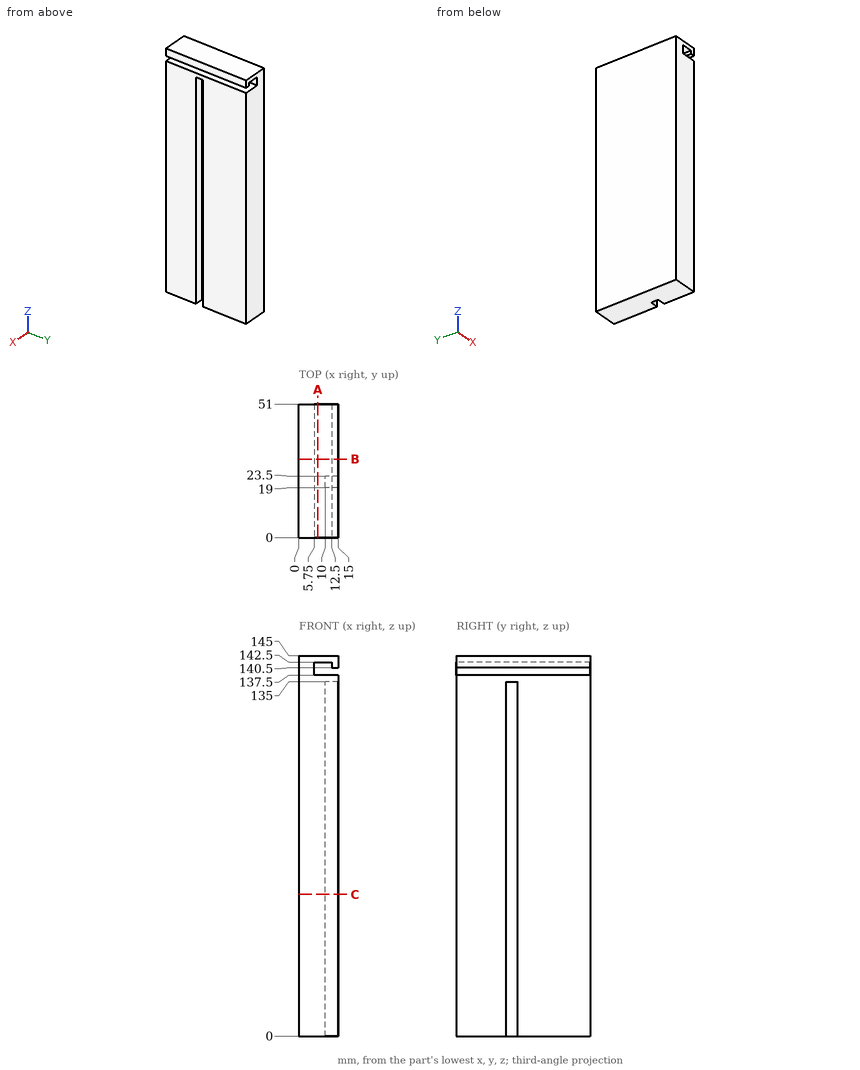
Verification items for this drawing (mm, ordinates from the low corner). Coordinates: 2 decimals unless noted, no trailing zeros. Write each loop counter-clockwise with the first axis right and the second up, starting at its lowest first coordinate (ties: lowest second). Pieces come first, ordered by that corner, then holes. Notation, with made-up numbers: M 45.25,85 L 94.25,85 A15 cw 94.25,91 Z; hole C -37,-23 d3. An arc over 180 degrees is marked long. One line per item, written item: value. Start each with the question number.
(1) Scan lines: line 1 along Z through (x, y) = (11.75, 44); line 2 along Y through (x, z) = (10.5, 32); line 3 along Z through (x, y) = (13.25, 15). Record each from-to range of solid material in increasing order. Write a range as [from, to].
(2) Sectioned sample at C-C, the plane z = 54. Enter the section's corners in (x, y), and give its area (4 significant figures).
(3) Sectioned sample at A-A, the plane x = 7.25. Enter the section's corners in (y, z), and give its area (3 significant figures).
(4) Sectioned sample at B-B, the plane y = 30. Enter the section's corners in (x, z), and give its area (3 significant figures).
Filled sheet:
1. line 1: [0, 137.5], [142.5, 145]
1. line 2: [0, 19], [23.5, 51]
1. line 3: [0, 137.5], [140.5, 145]
2. outline: M 0,0 L 15,0 L 15,19 L 10,19 L 10,23.5 L 15,23.5 L 15,51 L 0,51 Z
2. area: 742.5 mm²
3. outline: M 0,0 L 51,0 L 51,137.5 L 0,137.5 Z; M 0,142.5 L 51,142.5 L 51,145 L 0,145 Z
3. area: 7,140 mm²
4. outline: M 0,0 L 15,0 L 15,137.5 L 5.75,137.5 L 5.75,142.5 L 12.5,142.5 L 12.5,140.5 L 15,140.5 L 15,145 L 0,145 Z
4. area: 2,130 mm²
